For this review, take the finished solid that the model builds, in its own axes (mm). A direction names the side the tool comes from. Coordinates: 2 decimals unless noted, no trailing zeros. Write each loop counter-clockwise with the first axis right and the second up, starting at its lowest first coordinate (ties: lowest second). Pieces come first, ordered by that corner, then holes. Notation, with made-up numbers: M 36,26.25 L 80,26.25 A19 ccw 80,35.25 Z; hole C 49,82 d8. An arc over 180 degrees is marked long. One line per question, with ' | ' between items.
Autodesk Inventor part; units mm, degrees
ref_plane "YZ Plane" through (0, 0, 0) normal (1, 0, 0) x (0, 1, 0)
ref_plane "XZ Plane" through (0, 0, 0) normal (0, 1, 0) x (-1, 0, 0)
ref_plane "XY Plane" through (0, 0, 0) normal (0, 0, 1) x (1, 0, 0)
sketch "Sketch1" plane through (0, 0, 0) normal (1, 0, 0) x (0, 1, 0)
  line L0 (0, 11.5) -> (56, 11.5)
  line L1 (56, 11.5) -> (56, -11.5)
  line L2 (56, -11.5) -> (0, -11.5)
  line L3 (0, -11.5) -> (0, 11.5)
  point P0 (0, 0)
  dimension "d0" = 0
  dimension "d1" = 23
  dimension "d2" = 56
  dimension "d3" = 11.5
extrude "Extrusion1" add sketch "Sketch1" along normal mid plane 8
sketch "Sketch2" plane through (4, 0, 0) normal (1, 0, 0) x (0, 0, -1)
  line L0 (11.5, 56) -> (-11.5, 56)
  line L1 (-6.5, 56) -> (6.5, 56)
  line L2 (6.5, 56) -> (6.5, 43)
  line L3 (6.5, 43) -> (-6.5, 43)
  line L4 (-6.5, 43) -> (-6.5, 56)
  point P0 (0, 0)
  dimension "d6" = 13
  dimension "d7" = 13
  dimension "d8" = 6.5
extrude "Extrusion2" cut sketch "Sketch2" against normal through all
sketch "Sketch4" plane through (-4, 0, 11.5) normal (0, 0, 1) x (1, 0, 0)
  circle A0 centre (4, 51) radius 1.5
  line L0 (0, 56) -> (8, 56)
  line L1 (0, 0) -> (8, 0)
  point P0 (4, 0)
  point P1 (4, 0)
  dimension "d12" = 3
  dimension "d13" = 5
hole "Hole1" at (0, 51, 11.5) direction (0, 0, -1) diameter 3 end through all
sketch "Sketch5" plane through (-4, 0, -11.5) normal (0, -1, 0) x (1, 0, 0)
  circle A0 centre (4, 16.5) radius 1.5
  circle A1 centre (4, 6.5) radius 1.5
  point P0 (4, 11.5)
  dimension "d21" = 3
  dimension "d23" = 10
  dimension "d24" = 5
hole "Hole2" at (0, 0, 5) at (0, 0, -5) direction (0, 1, 0) diameter 2.459 depth 13 tip angle 118
properties part number "Gripper_Outer_Support_2" material "Aluminum 6061"
1. Take a section at B-B on y = 43.5. State the section outline as (x, z) points.
Computed values:
outline: M -4,-11.5 L 4,-11.5 L 4,-6.5 L -4,-6.5 Z; M -4,6.5 L 4,6.5 L 4,11.5 L -4,11.5 Z
2. Clearance check with a flat-ended pin moving along its axis: P1, Ø2.5, axis at x = 0, y = 51, coming from the +Z side. State where the tip first meets the part, or that it passes through.
Computed values:
P1: passes through
3. For line 1 along X through (y, z) = (51, 7.8); line 2 along X through (y, z) = (4.75, -5); line 3 along Z through (x, y) = (0, 3), list the stretches that pass through material, from the lowest coordinate up.
Computed values:
line 1: x = -4 to -1.5, 1.5 to 4 | line 2: x = -4 to -1.23, 1.23 to 4 | line 3: z = -11.5 to -6.23, -3.77 to 3.77, 6.23 to 11.5
4. Take a section at C-C on z = -7. State the section outline as (x, y) points.
Computed values:
outline: M -4,0 L 4,0 L 4,56 L -4,56 Z; hole C 0,51 d3
5. Take a section at A-A on y = 51. State the section outline as (x, z) points.
Computed values:
outline: M -4,-11.5 L -1.5,-11.5 L -1.5,-6.5 L -4,-6.5 Z; M -4,6.5 L -1.5,6.5 L -1.5,11.5 L -4,11.5 Z; M 1.5,-11.5 L 4,-11.5 L 4,-6.5 L 1.5,-6.5 Z; M 1.5,6.5 L 4,6.5 L 4,11.5 L 1.5,11.5 Z
6. Machinability: for faces 4 (the flat face through (0, 56, -9)), 5 (the cylindrical face through (-0.05, 6.59, 6.23)), 6 (the flat face through (0, 43, 0)), which of the approach directions +Z, -Z, +X, -X, +Y, -Y give a long, thin tool a straight path to every point of the face, cutting with its end or side? Answer none if there is none.
Computed values:
face 4: +Z, -Z, +X, -X, +Y | face 5: -Y | face 6: +X, -X, +Y
7. Take a section at D-D on x = 3. State the section outline as (y, z) points.
Computed values:
outline: M 0,-11.5 L 56,-11.5 L 56,-6.5 L 43,-6.5 L 43,6.5 L 56,6.5 L 56,11.5 L 0,11.5 Z
8. Draft analysis for pull direction X (two halves, no side actions). For faces 1 (the flat face through (4, 28, 0)), 2 (the flat face through (0, 49, 6.5)), 3 (the cylindrical face through (-0.07, 52.5, -9.04)), state which applies: pulls with the +X half, pulls with the -X half, needs draft (parallel to the pull), parting line crosses it, or undercut.
Computed values:
face 1: pulls with the +X half | face 2: needs draft | face 3: undercut
